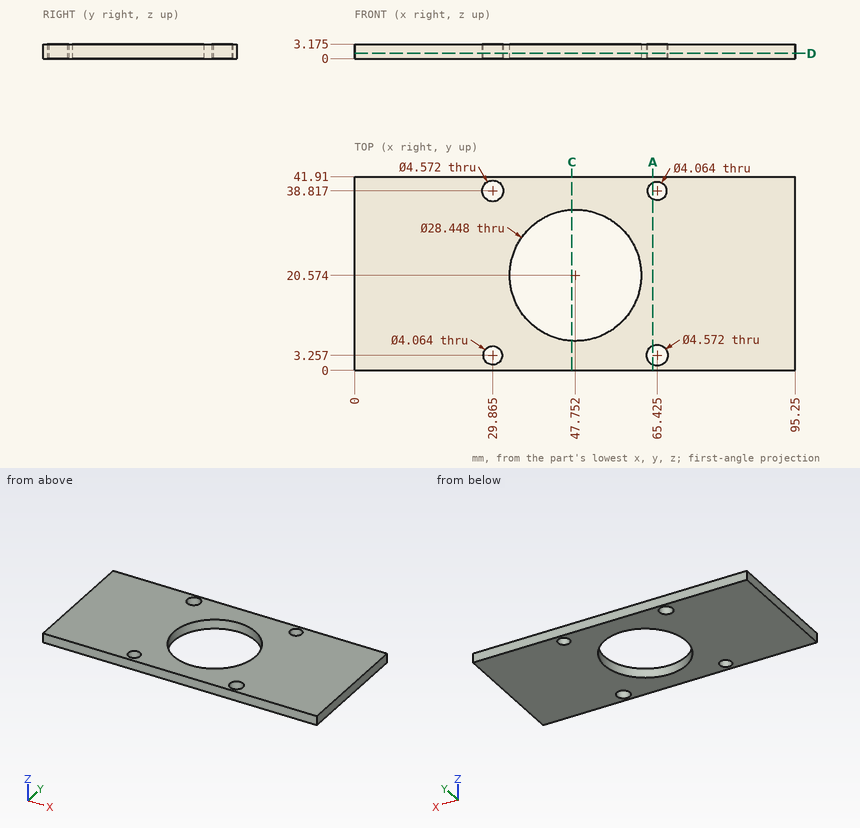
Print and shaded views of the part. All mm, measured from the part's lowest x, y and z. Round coordinates to 2 decimals unless told otherwise and drop trailing zeros. Write each loop counter-clockwise with the first axis right and the second up, starting at its lowest first coordinate (ties: lowest second). Pieces come first, ordered by that corner, then holes. Notation, with made-up numbers: (68, -39) -> (79, -39) arc R17 cw to (79, -31) -> close; hole circle Ø7 at (69, -38). An arc over 180 degrees is marked (long way). Write item = value, one per line.
(1) Probe L1, parallel to Y at x = 65.5, z = 3; L2, parallel to X at y = 39.5, z = 1; L3, parallel to X at y = 23, z = 0.3. List the from-to ranges inside material, lowest first.
Answer:
L1 = 0 to 0.97, 5.54 to 36.79, 40.85 to 41.91
L2 = 0 to 27.68, 32.05 to 63.51, 67.34 to 95.25
L3 = 0 to 33.74, 61.77 to 95.25
(2) Band-saw the part on C-C (x = 47). Give the cut face in (y, z) (1 decimal).
Answer:
outline = (0, 0) -> (6.4, 0) -> (6.4, 3.2) -> (0, 3.2) -> close; (34.8, 0) -> (41.9, 0) -> (41.9, 3.2) -> (34.8, 3.2) -> close
(3) Band-saw the part on A-A (x = 64.5). Give the cut face in (y, z) (1 decimal).
Answer:
outline = (0, 0) -> (1.2, 0) -> (1.2, 3.2) -> (0, 3.2) -> close; (5.3, 0) -> (37, 0) -> (37, 3.2) -> (5.3, 3.2) -> close; (40.6, 0) -> (41.9, 0) -> (41.9, 3.2) -> (40.6, 3.2) -> close
(4) Band-saw the part on D-D (z = 1.15). State how many separate pieces and enclosed holes the cut face has, then the cut area to 3 significant figures.
Answer:
separate_pieces = 1
enclosed_holes = 5
area = 3,300 mm2
